Design review of the part built by this model. Coordinates are the model's own, in mm. A direction names the side the tool comes from. Give positions to 0.01 mm unless a question says otherwise; leave off trailing zeros. Loops run counter-clockwise (first coordinate to the right, second up) from the corner with the lowest first, then second, coordinate; pieces in that order, holes last. Notation, with made-up numbers: (-34, -34) - (25, -34) arc R31 cw to (25, -10) - close; hole circle Ø4 at (80, -1). An arc over 180 degrees is marked (long way). Write each question's results on one line, items separated by ' | '.
```python
from build123d import *

# Parameters (mm, degrees)
SKETCH1_R           = 19.5
SKETCH1_R_2         = 14.5
BOSS_EXTRUDE1_DEPTH = 23.9
SKETCH2_R           = 38.1
SKETCH2_R_2         = 19.5
BOSS_EXTRUDE2_DEPTH = 3
SKETCH3_R           = 20
SKETCH3_R_2         = 19.5
BOSS_EXTRUDE3_DEPTH = 10
SKETCH4_R           = 19.5
SKETCH4_R_2         = 4.5
SKETCH4_R_3         = 1.125
BOSS_EXTRUDE4_DEPTH = 3


with BuildPart() as part:
    # Sketch1 → Boss-Extrude1 (new body)
    with BuildSketch(Plane(origin=(0, 0, 0), x_dir=(1, 0, 0), z_dir=(0, 1, 0))):
        Circle(SKETCH1_R)
        Circle(SKETCH1_R_2, mode=Mode.SUBTRACT)
    extrude(amount=BOSS_EXTRUDE1_DEPTH)

    # Sketch2 → Boss-Extrude2 (add)
    with BuildSketch(Plane.XZ):
        Circle(SKETCH2_R)
        Circle(SKETCH2_R_2, mode=Mode.SUBTRACT)
    extrude(amount=-BOSS_EXTRUDE2_DEPTH)

    # Sketch3 → Boss-Extrude3 (add)
    with BuildSketch(Plane(origin=(0, 3, 0), x_dir=(1, 0, 0), z_dir=(0, 1, 0))):
        Circle(SKETCH3_R)
        Circle(SKETCH3_R_2, mode=Mode.SUBTRACT)
    extrude(amount=BOSS_EXTRUDE3_DEPTH)

    # Sketch4 → Boss-Extrude4 (add)
    with BuildSketch(Plane(origin=(0, 23.9, 0), x_dir=(1, 0, 0), z_dir=(0, 1, 0))):
        Circle(SKETCH4_R)
        Circle(SKETCH4_R_2, mode=Mode.SUBTRACT)
        with Locations((0, 6)):
            Circle(SKETCH4_R_3, mode=Mode.SUBTRACT)
        with Locations((6, 0)):
            Circle(SKETCH4_R_3, mode=Mode.SUBTRACT)
        with Locations((0, -6)):
            Circle(SKETCH4_R_3, mode=Mode.SUBTRACT)
        with Locations((-6, 0)):
            Circle(SKETCH4_R_3, mode=Mode.SUBTRACT)
    extrude(amount=BOSS_EXTRUDE4_DEPTH)


solid = part.part
```
Item 1: Draft analysis for pull direction X (two halves, no side actions). For faces 1 (the face through (-3.4, 23.9, -3.4)), 2 (the face through (4.876, 25.379, -0.049)), 3 (the face through (16, 0, 1)), 4 (the face through (-2.539, 19.853, -19.334)), state which applies: +X half, -X half, draft (parallel to the pull), parting line (faces both ways), or undercut.
Output values:
face 1: undercut | face 2: undercut | face 3: draft | face 4: parting line
Item 2: We need section C-C on y = 16.5. Give the boundary of the cut face in (x, z), then the cut area to 3 significant figures.
Output values:
outline: circle Ø39 at (0, 0); hole circle Ø29 at (0, 0) | area: 534 mm²
Item 3: Wall thickness on probe 1 along Z at (x, y) = (0, 26.3) (3 decimals); probe 2 along X at (y, z) = (6, 0); probe 3 along X at (y, z) = (15, 0): over which ranges is each line inside the solid? List them lowest first.
Output values:
probe 1: z = -19.5 to -7.125, -4.875 to -4.5, 4.5 to 4.875, 7.125 to 19.5 | probe 2: x = -20 to -14.5, 14.5 to 20 | probe 3: x = -19.5 to -14.5, 14.5 to 19.5
Item 4: Clearance check with flat-ended pins moving along their axes: P1, Ø8.5, axis at x = -7, z = -3.5, coming from the -Y side; P2, Ø1.5, axis at x = 8, y = 18.5, coming from the -Z side; P3, Ø2, axis at x = 17, y = 11.5, coming from the -Z side. State where each tip first meets the part, or that it passes through.
Output values:
P1: stops at y = 23.9 | P2: stops at z = -18.1 | P3: stops at z = -12
Item 5: We need section D-D on z = -27.5. Give the boundary of the cut face in (x, y).
Output values:
outline: (-26.37, 0) - (26.37, 0) - (26.37, 3) - (-26.37, 3) - close
Item 6: We need section B-B on z = 0. Give the boundary of the cut face in (x, y) (3 decimals).
Output values:
outline: (-38.1, 0) - (-14.5, 0) - (-14.5, 23.9) - (-7.125, 23.9) - (-7.125, 26.9) - (-19.5, 26.9) - (-19.5, 13) - (-20, 13) - (-20, 3) - (-38.1, 3) - close; (-4.875, 23.9) - (-4.5, 23.9) - (-4.5, 26.9) - (-4.875, 26.9) - close; (4.5, 23.9) - (4.875, 23.9) - (4.875, 26.9) - (4.5, 26.9) - close; (7.125, 23.9) - (14.5, 23.9) - (14.5, 0) - (38.1, 0) - (38.1, 3) - (20, 3) - (20, 13) - (19.5, 13) - (19.5, 26.9) - (7.125, 26.9) - close
Item 7: Tool access review of faces 5 (the face through (6.691, 11.783, 12.864)), 6 (the face through (-0.59, 25.38, -4.46)), 7 (the face through (19.2, 13, 4.4)): name each direction out of +Z, -Z, +X, -X, +Y, -Y from which nothing blocks a thin tool from reaching the whole face with its end or side.
Output values:
face 5: -Y | face 6: +Y, -Y | face 7: +Y
Item 8: We need section A-A on x = 0. Give the boundary of the cut face in (y, z) (3 decimals), then the cut area to 3 significant figures.
Output values:
outline: (0, -38.1) - (3, -38.1) - (3, -20) - (13, -20) - (13, -19.5) - (26.9, -19.5) - (26.9, -7.125) - (23.9, -7.125) - (23.9, -14.5) - (0, -14.5) - close; (0, 14.5) - (23.9, 14.5) - (23.9, 7.125) - (26.9, 7.125) - (26.9, 19.5) - (13, 19.5) - (13, 20) - (3, 20) - (3, 38.1) - (0, 38.1) - close; (23.9, -4.875) - (26.9, -4.875) - (26.9, -4.5) - (23.9, -4.5) - close; (23.9, 4.5) - (26.9, 4.5) - (26.9, 4.875) - (23.9, 4.875) - close | area: 437 mm²
